from build123d import *

# Parameters (mm, degrees)
SKETCH1_R               = 37.5
SKETCH1_R_2             = 2.3
BOSS_EXTRUDE1_DEPTH     = 2
SKETCH2_R               = 37.5
SKETCH2_R_2             = 4.5
BOSS_EXTRUDE2_DEPTH     = 5
BOSS_EXTRUDE3_DEPTH     = 5
SKETCH4_R               = 17.5
CUT_EXTRUDE1_DEPTH      = 7
CUT_EXTRUDE2_DEPTH      = 7
CUT_EXTRUDE2_DEPTH_BACK = 2.5
CUT_EXTRUDE4_DEPTH      = 3
CUT_EXTRUDE4_DEPTH_BACK = 2.5
SKETCH10_R              = 1.65
CUT_EXTRUDE7_DEPTH      = 20
SKETCH9_R               = 1.65
CUT_EXTRUDE6_DEPTH      = 20
CUT_EXTRUDE8_DEPTH      = 4
FILLET1_R               = 3


with BuildPart() as part:
    # Sketch1 → Boss-Extrude1 (new body)
    with BuildSketch(Plane(origin=(0, 0, 0), x_dir=(1, 0, 0), z_dir=(0, 1, 0))):
        Circle(SKETCH1_R)
        with Locations((0, 27.5)):
            Circle(SKETCH1_R_2, mode=Mode.SUBTRACT)
        with Locations((23.815698604, 13.75)):
            Circle(SKETCH1_R_2, mode=Mode.SUBTRACT)
        with Locations((23.815698604, -13.75)):
            Circle(SKETCH1_R_2, mode=Mode.SUBTRACT)
        with Locations((0, -27.5)):
            Circle(SKETCH1_R_2, mode=Mode.SUBTRACT)
        with Locations((-23.815698604, -13.75)):
            Circle(SKETCH1_R_2, mode=Mode.SUBTRACT)
        with Locations((-23.815698604, 13.75)):
            Circle(SKETCH1_R_2, mode=Mode.SUBTRACT)
    extrude(amount=BOSS_EXTRUDE1_DEPTH)

    # Sketch2 → Boss-Extrude2 (add)
    with BuildSketch(Plane(origin=(0, 2, 0), x_dir=(1, 0, 0), z_dir=(0, 1, 0))):
        Circle(SKETCH2_R)
        with Locations((-23.815698604, 13.75)):
            Circle(SKETCH2_R_2, mode=Mode.SUBTRACT)
        with Locations((-23.815698604, -13.75)):
            Circle(SKETCH2_R_2, mode=Mode.SUBTRACT)
        with Locations((0, -27.5)):
            Circle(SKETCH2_R_2, mode=Mode.SUBTRACT)
        with Locations((23.815698604, -13.75)):
            Circle(SKETCH2_R_2, mode=Mode.SUBTRACT)
        with Locations((23.815698604, 13.75)):
            Circle(SKETCH2_R_2, mode=Mode.SUBTRACT)
        with Locations((0, 27.5)):
            Circle(SKETCH2_R_2, mode=Mode.SUBTRACT)
    extrude(amount=BOSS_EXTRUDE2_DEPTH)

    # Sketch3 → Boss-Extrude3 (add)
    with BuildSketch(Plane(origin=(0, 7, 0), x_dir=(1, 0, 0), z_dir=(0, 1, 0))):
        with BuildLine():
            Line((-26.527052262, 26.50595213), (-12.379291055, 12.369444327))
            ThreePointArc((-12.379291055, 12.369444327), (-8.756029172, 15.151962023), (-4.536058371, 16.901898546))
            Line((-4.536058371, 16.901898546), (-9.720125081, 36.218354027))
            ThreePointArc((-9.720125081, 36.218354027), (-18.762919655, 32.468490048), (-26.527052262, 26.50595213))
        make_face()
        with BuildLine():
            ThreePointArc((-16.901898546, -4.536058371), (-17.499998615, -0.006962688), (-16.905502698, 4.52260749))
            Line((-16.905502698, 4.52260749), (-36.226077211, 9.691301765))
            ThreePointArc((-36.226077211, 9.691301765), (-37.499997032, -0.014920046), (-36.218354027, -9.720125081))
            Line((-36.218354027, -9.720125081), (-16.901898546, -4.536058371))
        make_face()
        with BuildLine():
            ThreePointArc((4.52260749, 16.905502698), (8.743969443, 15.158924711), (12.369444327, 12.379291055))
            Line((12.369444327, 12.379291055), (26.50595213, 26.527052262))
            ThreePointArc((26.50595213, 26.527052262), (18.737077377, 32.483410095), (9.691301765, 36.226077211))
            Line((9.691301765, 36.226077211), (4.52260749, 16.905502698))
        make_face()
        with BuildLine():
            ThreePointArc((16.901898546, 4.536058371), (17.499998615, 0.006962688), (16.905502698, -4.52260749))
            Line((16.905502698, -4.52260749), (36.226077211, -9.691301765))
            ThreePointArc((36.226077211, -9.691301765), (37.499997032, 0.014920046), (36.218354027, 9.720125081))
            Line((36.218354027, 9.720125081), (16.901898546, 4.536058371))
        make_face()
        with BuildLine():
            Line((-12.805791077, -12.81598516), (-26.50595213, -26.527052262))
            ThreePointArc((-26.50595213, -26.527052262), (-18.737077377, -32.483410095), (-9.691301765, -36.226077211))
            Line((-9.691301765, -36.226077211), (-4.682147808, -17.501864262))
            Line((-4.682147808, -17.501864262), (-12.805791077, -12.81598516))
        make_face()
        with BuildLine():
            Line((12.819708432, -12.809511387), (4.694715176, -17.493072864))
            Line((4.694715176, -17.493072864), (9.720125081, -36.218354027))
            ThreePointArc((9.720125081, -36.218354027), (18.762919655, -32.468490048), (26.527052262, -26.50595213))
            Line((26.527052262, -26.50595213), (12.819708432, -12.809511387))
        make_face()
    extrude(amount=BOSS_EXTRUDE3_DEPTH)

    # Sketch4 → Cut-Extrude1 (cut)
    with BuildSketch(Plane(origin=(0, 7, 0), x_dir=(1, 0, 0), z_dir=(0, 1, 0))):
        Circle(SKETCH4_R)
    extrude(amount=-CUT_EXTRUDE1_DEPTH, mode=Mode.SUBTRACT)

    # Sketch5 → Cut-Extrude2 (cut, two sides)
    with BuildSketch(Plane(origin=(-8.743969443, 0, 15.158924711), x_dir=(-0.866224269, 0, -0.499655397), z_dir=(0.499655397, 0, -0.866224269))) as cut_extrude2_sk:
        with BuildLine():
            Line((1.5, 7), (3.290896534, 7))
            Line((3.290896534, 7), (1.645448267, 9.85))
            Line((1.645448267, 9.85), (-1.645448267, 9.85))
            Line((-1.645448267, 9.85), (-3.290896534, 7))
            Line((-3.290896534, 7), (-1.5, 7))
            ThreePointArc((-1.5, 7), (0, 8.5), (1.5, 7))
        make_face()
        with BuildLine():
            Line((1.645448267, 4.15), (3.290896534, 7))
            Line((3.290896534, 7), (1.5, 7))
            ThreePointArc((1.5, 7), (0, 5.5), (-1.5, 7))
            Line((-1.5, 7), (-3.290896534, 7))
            Line((-3.290896534, 7), (-1.645448267, 4.15))
            Line((-1.645448267, 4.15), (1.645448267, 4.15))
        make_face()
        with BuildLine():
            ThreePointArc((-1.5, 7), (0, 5.5), (1.5, 7))
            Line((1.5, 7), (0, 7))
            Line((0, 7), (-1.5, 7))
        make_face()
        with BuildLine():
            Line((0, 7), (1.5, 7))
            ThreePointArc((1.5, 7), (0, 8.5), (-1.5, 7))
            Line((-1.5, 7), (0, 7))
        make_face()
    extrude(amount=CUT_EXTRUDE2_DEPTH, mode=Mode.SUBTRACT)
    extrude(cut_extrude2_sk.sketch, amount=-CUT_EXTRUDE2_DEPTH_BACK, mode=Mode.SUBTRACT)

    # Sketch7 → Cut-Extrude4 (cut, two sides)
    with BuildSketch(Plane(origin=(8.739633736, 0, 15.161424807), x_dir=(-0.866367132, 0, 0.499407642), z_dir=(-0.499407642, 0, -0.866367132))) as cut_extrude4_sk:
        Polygon((0, 7), (3.270607135, 7), (1.625158868, 9.85), (-1.665737666, 9.85), (-3.311185933, 7), (-0.020289399, 7), align=None)
        Polygon((1.625158868, 4.15), (3.270607135, 7), (0, 7), (-0.020289399, 7), (-3.311185933, 7), (-1.665737666, 4.15), align=None)
    extrude(amount=CUT_EXTRUDE4_DEPTH, mode=Mode.SUBTRACT)
    extrude(cut_extrude4_sk.sketch, amount=-CUT_EXTRUDE4_DEPTH_BACK, mode=Mode.SUBTRACT)

    # Sketch10 → Cut-Extrude7 (cut)
    with BuildSketch(Plane(origin=(8.739633736, 0, 15.161424807), x_dir=(-0.866367132, 0, 0.499407642), z_dir=(-0.499407642, 0, -0.866367132))):
        with Locations((-0.020289399, 7)):
            Circle(SKETCH10_R)
    extrude(amount=-CUT_EXTRUDE7_DEPTH, mode=Mode.SUBTRACT)

    # Sketch9 → Cut-Extrude6 (cut)
    with BuildSketch(Plane(origin=(-9.993107934, 0, 17.324485384), x_dir=(-0.866224269, 0, -0.499655397), z_dir=(0.499655397, 0, -0.866224269))):
        with Locations((0, 6.9)):
            Circle(SKETCH9_R)
    extrude(amount=-CUT_EXTRUDE6_DEPTH, mode=Mode.SUBTRACT)

    # Sketch14 → Cut-Extrude8 (cut)
    with BuildSketch(Plane.XZ):
        with BuildLine():
            Line((8.75, -15.155444566), (18.75, -32.475952642))
            ThreePointArc((18.75, -32.475952642), (20.878012246, -31.150579524), (22.912712953, -29.685982974))
            Line((22.912712953, -29.685982974), (12.715381935, -12.023687548))
            ThreePointArc((12.715381935, -12.023687548), (10.846318772, -13.733439813), (8.75, -15.155444566))
        make_face()
        with BuildLine():
            Line((4.055127897, -17.023687548), (14.252458915, -34.685982974))
            ThreePointArc((14.252458915, -34.685982974), (16.538187087, -33.656178747), (18.75, -32.475952642))
            Line((18.75, -32.475952642), (8.75, -15.155444566))
            ThreePointArc((8.75, -15.155444566), (6.470348373, -16.259907501), (4.055127897, -17.023687548))
        make_face()
    extrude(amount=-CUT_EXTRUDE8_DEPTH, mode=Mode.SUBTRACT)

    # Fillet1
    fillet1_edges = [part.edges().sort_by_distance(p)[0] for p in [
        (17.814047444, 4, -20.854835261),
        (9.153793406, 4, -25.854835261),
    ]]
    fillet(fillet1_edges, radius=FILLET1_R)


solid = part.part
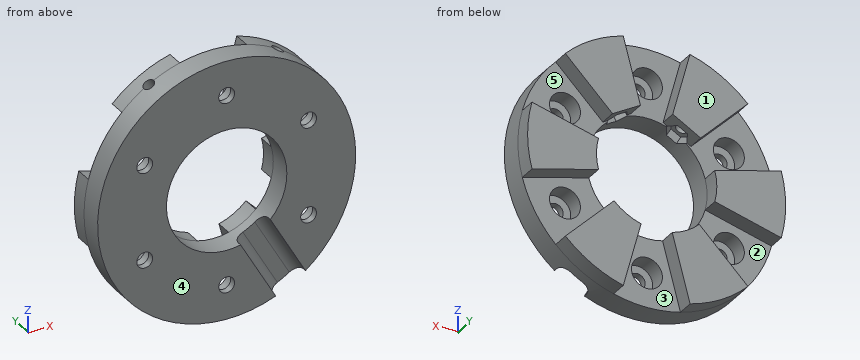
Can you work these out from the model? Positions are in its coordinate system, mm. Face numbers are marked on the shaded views. A direction names the side the tool comes from. Coordinates: 2 decimals unless noted, no trailing zeros. Write each loop counter-clockwise with the first axis right and the second up, starting at its lowest first coordinate (ties: lowest second). Pieces come first, ordered by that corner, then holes. Notation, with made-up numbers: (-40, 64.5) -> (-20, 64.5) arc R34 cw to (-20, 100.5) -> close; hole circle Ø3 at (57, 3.5). An arc over 180 degrees is marked (long way). Answer as CSV lines item,"result".
1) If we section it at C-C on z = 27.5: Count the separate pieces of the cut face and the enclosed holes in it, then the cut area to 3 significant figures.
Check result:
separate pieces,"2"
enclosed holes,"2"
area,"464 mm²"
2) If I drill on line 1 (Z direction, x = 0, y = 5.35); line 2 (Z direction, x = 0, y = 1.25); line 3 (X direction, y = 3.2, z = -13.75), over which ranges is the centre line in solid material (lowest first)? Write a range as from..to.
Check result:
line 1,"-37.5..-32, -23..-17.5, 17.5..23, 32..37.5"
line 2,"-37.5..-29.8, -25.2..-17.5, 17.5..25.2, 29.8..37.5"
line 3,"-34.89..-28.32, -19.32..-10.83, 12.6..19.32, 28.32..34.89"
3) If we mould it in two halves opening along Z, with no side actions, what happens to the marked faces 4 and 5? For each: +Z half, -Z half, draft (parallel to the pull), parting line (faces both ways), or undercut.
Check result:
face 4,"draft"
face 5,"undercut"
4) On a 3-axis mill with a long thin cutter (end or side, diameter ignored), from which of +Z, -Z, +X, -X, +Y, -Y can I reach the whole of each face in a straight line? I mean the marked faces 1, 2 and 3. Say none if no direction works.
Check result:
face 1,"+Z, -Z, +X, -X, +Y"
face 2,"+Y"
face 3,"-Z, +Y"
5) If we section it at B-B on z = 6: Please give me the cut outline in (x, y), then the cut area to 3 significant figures.
Check result:
outline,"(-37.02, 0) -> (-16.44, 0) -> (-16.44, 7) -> (-22.36, 7) -> (-22.36, 12) -> (-37.02, 12) -> close; (16.44, 0) -> (37.02, 0) -> (37.02, 12) -> (22.43, 12) -> (22.43, 7) -> (16.44, 7) -> close"
area,"434 mm²"
6) If we section it at A-A on x = 0: Please give me the cut outline in (y, z), then the cut area to 3 significant figures.
Check result:
outline,"(0, -37.5) -> (7, -37.5) -> (7, -32) -> (2, -32) -> (2, -29.8) -> (0, -29.8) -> close; (0, -25.2) -> (2, -25.2) -> (2, -23) -> (7, -23) -> (7, -17.5) -> (0, -17.5) -> close; (0, 17.5) -> (7, 17.5) -> (7, 23) -> (2, 23) -> (2, 25.2) -> (0, 25.2) -> close; (0, 29.8) -> (2, 29.8) -> (2, 32) -> (7, 32) -> (7, 37.5) -> (0, 37.5) -> close"
area,"172 mm²"
7) Will these pins go through, and if not, where does the flat tip stop? P1, Ø6, axis at x = 9.5, z = 14, coming from the -Y side; P2, Ø1.5, axis at y = 4.5, z = -21.5, coming from the -X side; P3, Ø7.5, axis at x = 23.82, z = -13.75, coming from the +Y side; P4, Ø3, axis at y = 3.5, z = -28.5, coming from the -X side.
Check result:
P1,"y = 0"
P2,"x = -31.24"
P3,"y = 2"
P4,"x = -26.02"
